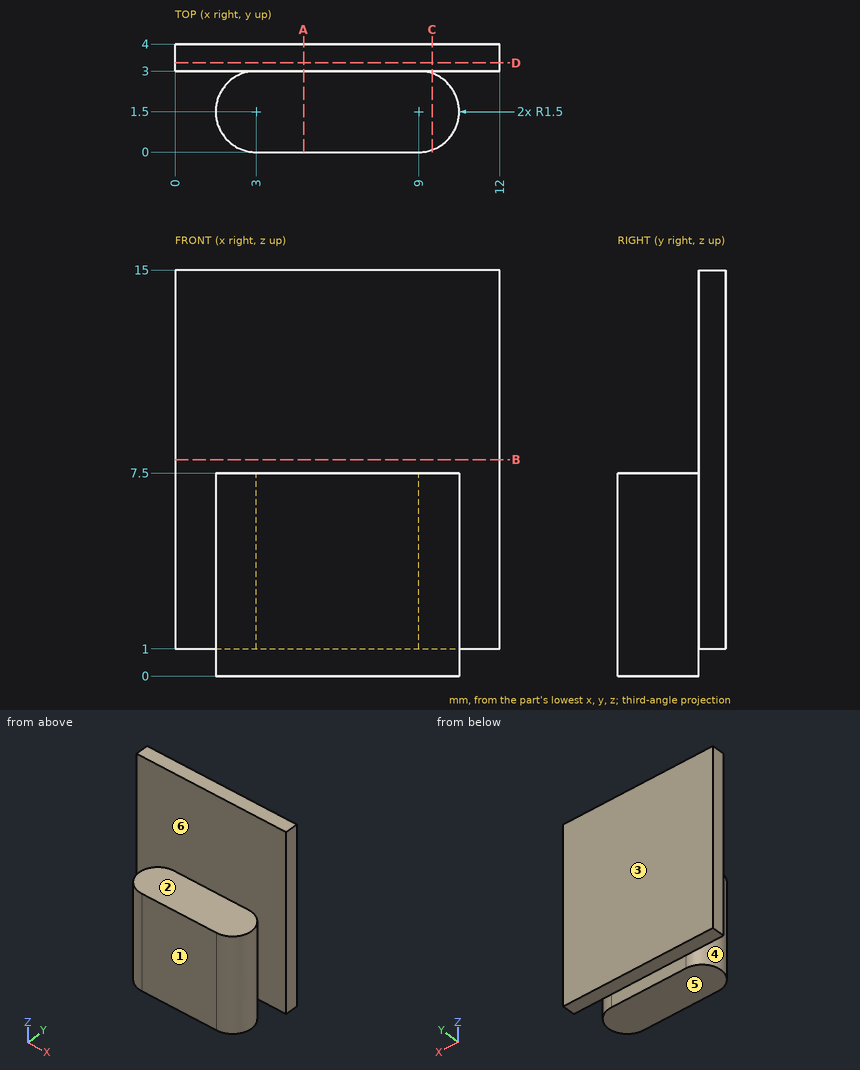
The figure shows three views and two pictorial views of one solid part (mm, origin at its lowest corner). Answer the questions. A direction names the side the tool comes from. Round coordinates to 2 decimals unless told otherwise and drop trailing zeros. Order: outer loops, then holes, each group sorted by start corner. A loop starts at its lowest first (then second) coordinate and runs counter-clockwise, first axis right, second up. Notation, with made-up numbers: M 65,-24.5 L 81,-24.5 A12 ccw 81,-19.5 Z; hole C 72.5,89 d11. An arc over 180 degrees is marked long. Put each result on its own line as item: value. Start each with the question number.
Q1. Flat-ended cylindrical pins translate along their axes: pin 1 (1 mm diameter, centred on x = 5, z = 9, fed in from -Y); pin 2 (1 mm diameter, centred on y = 1, z = 5, fed in from +X); pin 3 (0.8 mm diameter, centred on x = 5, z = 0.5, fed in from +Y). Find the tip coordinate at first contact, or state that the pin passes through.
Q2. Section B-B, the plane z = 8 is taken. Write down the section's boundary in (x, y), and give its area (3 significant figures).
Q3. A tool of negligible diameter and unlimited length cuts with its end or side. For the marked faces 1 and 2, from which of +Z, -Z, +X, -X, +Y, -Y can it reach the whole face along a straight path? Write none if from no direction.
Q4. Section C-C, the plane x = 9.5 is taken. Write down the section's boundary in (y, z).
Q5. Section A-A, the plane x = 4.75 is taken. Write down the section's boundary in (y, z), and give its area (3 significant figures).
Q6. Section D-D, the plane y = 3.3 is taken. Write down the section's boundary in (x, z).
Q7. Straight lines are drawn through the part: L1, parallel to Z at x = 10, y = 0.9; L2, parallel to Y at x = 3.75, z = 10.25; L3, parallel to Y at x = 2.25, z = 4. For each, find the intervals that lie inside material, in ascending order. Write a range as [from, to].
Q8. For a pull along Y with two mould halves and no side action, classify the marked faces 3, 4, 5 and 6 as pulls with the +Y half, pulls with the -Y half, needs draft (parallel to the pull), parting line crosses it, or undercut.
Findings below:
1. pin 1: stops at y = 3
1. pin 2: stops at x = 10.5
1. pin 3: stops at y = 3
2. outline: M 0,3 L 12,3 L 12,4 L 0,4 Z
2. area: 12.0 mm^2
3. face 1: +Z, -Z, +X, -X, -Y
3. face 2: +Z, +X, -X, -Y
4. outline: M 0.09,0 L 2.91,0 L 2.91,7.5 L 0.09,7.5 Z; M 3,1 L 4,1 L 4,15 L 3,15 Z
5. outline: M 0,0 L 3,0 L 3,1 L 4,1 L 4,15 L 3,15 L 3,7.5 L 0,7.5 Z
5. area: 36.5 mm^2
6. outline: M 0,1 L 12,1 L 12,15 L 0,15 Z
7. L1: z = [0, 7.5]
7. L2: y = [3, 4]
7. L3: y = [0.2, 2.8], [3, 4]
8. face 3: pulls with the +Y half
8. face 4: undercut
8. face 5: needs draft
8. face 6: undercut
